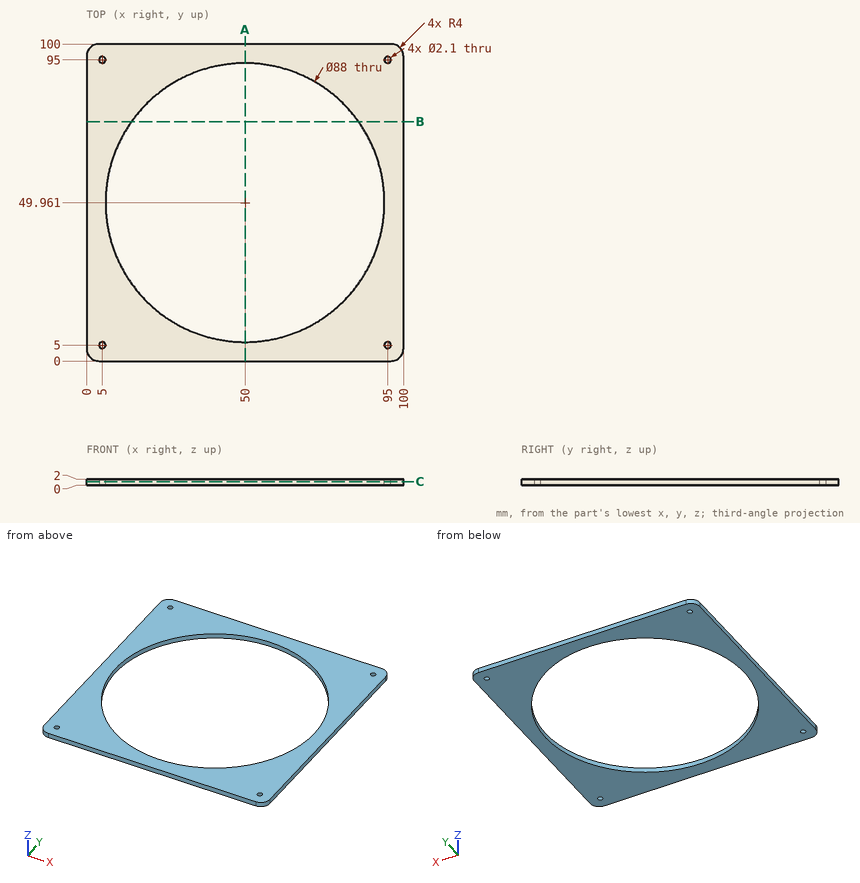
Source: three-view drawing plus pictorial views. Frame: mm from the lowest corner of the part. Give positions to 0.01 mm unless a question says otherwise; leave off trailing zeros. Write each loop counter-clockwise with the first axis right and the second up, starting at its lowest first coordinate (ties: lowest second). Pieces come first, ordered by that corner, then holes.
(1) Cut plane C-C, the plane z = 1.15. Return loops of the section in (x, y).
(2) Ray query, line 1 (Y direction, x = 95, z = 0.9); line 2 (Y direction, x = 51, z = 1); line 3 (Y direction, x = 50, z = 1). Return the intervals inside material, ascending.
(3) Cut plane A-A, the plane x = 50. Return loops of the section in (y, z).
(4) First-contact query: P1, Ø6, axis at x = 12, y = 55, coming from the +Z side; P2, Ø2.5, axis at x = 5, y = 95, coming from the -Z side. Flat tips, straight axial feed; report the tip coordinate or a pass-through.
(5) Cut plane B-B, the plane y = 75.5. Return loops of the section in (x, z).
Values follow:
1. outline: (0, 4) arc R4 ccw to (4, 0) - (96, 0) arc R4 ccw to (100, 4) - (100, 96) arc R4 ccw to (96, 100) - (4, 100) arc R4 ccw to (0, 96) - close; hole circle Ø2.1 at (5, 5); hole circle Ø2.1 at (5, 95); hole circle Ø88 at (50, 49.96); hole circle Ø2.1 at (95, 5); hole circle Ø2.1 at (95, 95)
2. line 1: y = 0 to 3.95, 6.05 to 93.95, 96.05 to 100
2. line 2: y = 0 to 5.97, 93.95 to 100
2. line 3: y = 0 to 5.96, 93.96 to 100
3. outline: (0, 0) - (5.96, 0) - (5.96, 2) - (0, 2) - close; (93.96, 0) - (100, 0) - (100, 2) - (93.96, 2) - close
4. P1: passes through
4. P2: stops at z = 0
5. outline: (0, 0) - (14.17, 0) - (14.17, 2) - (0, 2) - close; (85.83, 0) - (100, 0) - (100, 2) - (85.83, 2) - close
